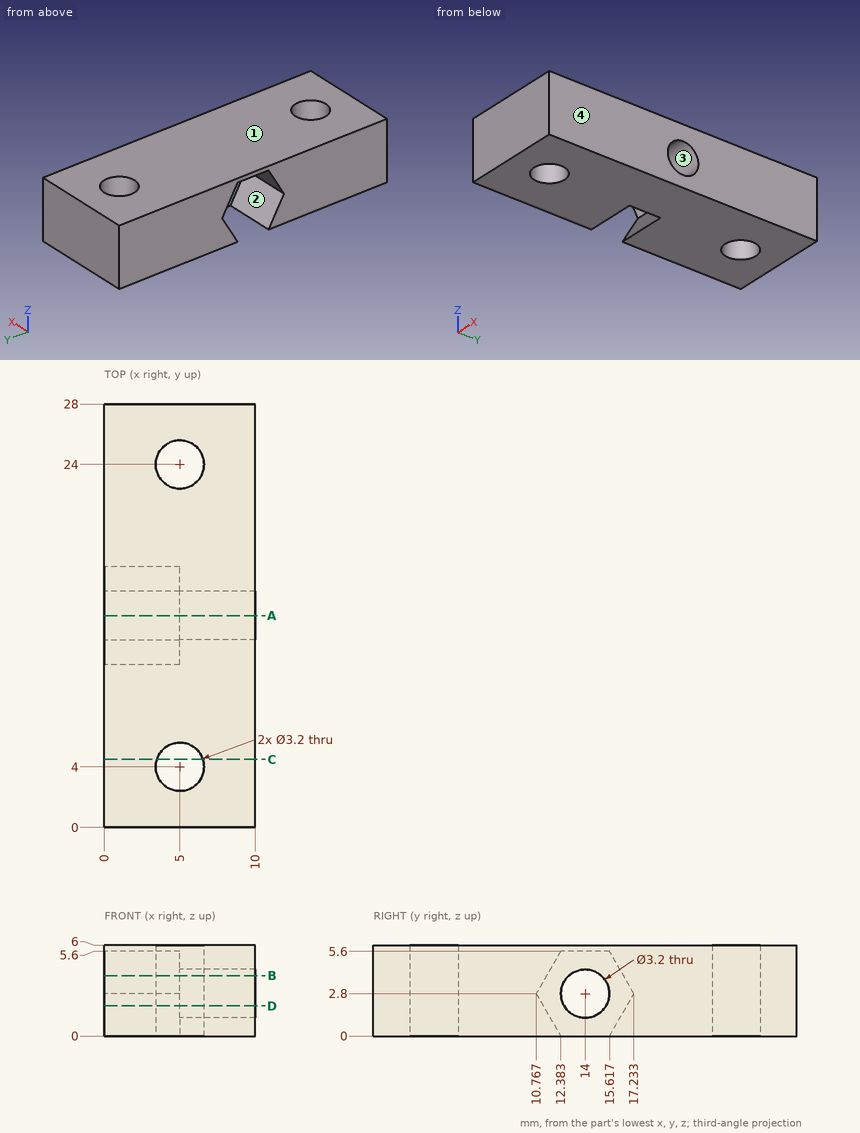
Job drawing, mm, ordinate dimensions from the low corner. One solid piece. Give positions to 0.01 mm unless a question says otherwise; leave off trailing zeros. Write each loop counter-clockwise with the first axis right and the second up, starting at its lowest first coordinate (ties: lowest second). Pieces come first, ordered by that corner, then holes. Notation, with made-up numbers: M 40.25,10 L 56.25,10 A19 cw 56.25,42 Z; hole C 44,71.5 d5. An arc over 180 degrees is marked long. Put each result on its own line as item: value. Start each with the question number.
(1) Probe L1, parallel to X at y = 4, z = 4.1; L2, parallel to Z at x = 7.45, y = 14; L3, parallel to Y at x = 2, z = 1.75. List the from-to ranges inside material, lowest first.
(2) Mould opens along Z. For the marked faces 1, 2, 3 and 4 say: +Z half, -Z half, draft (parallel to the pull), parting line (faces both ways), or undercut.
(3) Band-saw the part on D-D, the plane z = 2. Write the cut outline in (x, y) (1 decimal).
(4) Band-saw the part on C-C, the plane y = 4.5. Write the cut outline in (x, z).
(5) Flat gauge pin, fed straight in: pin 1 Ø1.6 at (x, y) = (3, 13.5) entering from -Z. Where does the tip first touch, or does it go through?
(6) Band-saw the part on A-A, the plane y = 14. Write the cut outline in (x, z).
(7) Band-saw the part on B-B, the plane z = 4. Write the cut outline in (x, y), and give its area (3 significant figures).
Response values:
1. L1: x = 0 to 3.4, 6.6 to 10
1. L2: z = 0 to 1.2, 4.4 to 6
1. L3: y = 0 to 11.37, 16.63 to 28
2. face 1: +Z half
2. face 2: undercut
2. face 3: undercut
2. face 4: draft
3. outline: M 0,0 L 10,0 L 10,12.6 L 5,12.6 L 5,11.2 L 0,11.2 Z; M 0,16.8 L 5,16.8 L 5,15.4 L 10,15.4 L 10,28 L 0,28 Z; hole C 5,4 d3.2; hole C 5,24 d3.2
4. outline: M 0,0 L 3.48,0 L 3.48,6 L 0,6 Z; M 6.52,0 L 10,0 L 10,6 L 6.52,6 Z
5. pin 1: stops at z = 5.6
6. outline: M 0,5.6 L 5,5.6 L 5,4.4 L 10,4.4 L 10,6 L 0,6 Z; M 5,0 L 10,0 L 10,1.2 L 5,1.2 Z
7. outline: M 0,0 L 10,0 L 10,12.94 L 5,12.94 L 5,11.46 L 0,11.46 Z; M 0,16.54 L 5,16.54 L 5,15.06 L 10,15.06 L 10,28 L 0,28 Z; hole C 5,4 d3.2; hole C 5,24 d3.2
7. area: 228 mm2
